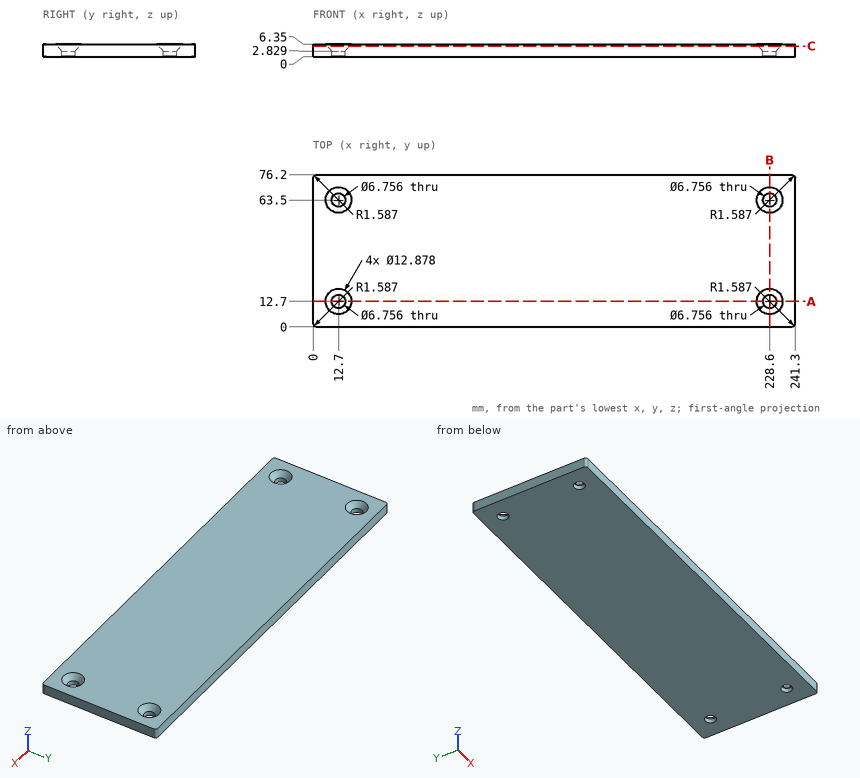
The drawing under review shows one solid part. Ordinate dimensions are in mm from its lowest x, y, z. Coordinates: 2 decimals unless noted, no trailing zeros. Write each loop counter-clockwise with the first axis right and the second up, starting at its lowest first coordinate (ties: lowest second). Pieces come first, ordered by that corner, then holes. Notation, with made-up numbers: (35.5, 37) -> (85.5, 37) arc R21 ccw to (85.5, 59) -> close; hole circle Ø3 at (-37, -26). An arc over 180 degrees is marked (long way). Write each question's results on one line, items separated by ' | '. Start each with the question number.
1) Wall thickness on L1, parallel to X at y = 63.5, z = 1.8; L2, parallel to X at y = 10.5, z = 1.25 (1 decimal); L3, parallel to Z at x = 225, y = 65: over which ranges is each line inside the solid? List them lowest first. Write a range as [from, to].
2) Consider section B-B (x = 228.6). Write out the cut boundary in (y, z).
3) Consider section C-C (z = 5.25). Write out the cut boundary in (x, y) (1 decimal).
4) Consider section A-A (y = 12.7). Write out the cut boundary in (x, z).
5) Insertion check: pin 1 (5.5 mm diameter, centred on x = 228.6, y = 12.7, fed in from -Z); pin 2 (9 mm diameter, centred on x = 12.7, y = 12.7, fed in from +Z). Each pin has a flat end and moves straight along its axis. Give the tip position at first contact, or say it passes through.
Geometry says:
1) L1: [0, 9.32], [16.08, 225.22], [231.98, 241.3] | L2: [0, 10.1], [15.3, 226], [231.2, 241.3] | L3: [0, 3.43]
2) outline: (0, 0) -> (9.32, 0) -> (9.32, 2.83) -> (6.26, 6.35) -> (0, 6.35) -> close; (16.08, 0) -> (60.12, 0) -> (60.12, 2.83) -> (57.06, 6.35) -> (19.14, 6.35) -> (16.08, 2.83) -> close; (66.88, 0) -> (76.2, 0) -> (76.2, 6.35) -> (69.94, 6.35) -> (66.88, 2.83) -> close
3) outline: (0, 1.6) arc R1.6 ccw to (1.6, 0) -> (239.7, 0) arc R1.6 ccw to (241.3, 1.6) -> (241.3, 74.6) arc R1.6 ccw to (239.7, 76.2) -> (1.6, 76.2) arc R1.6 ccw to (0, 74.6) -> close; hole circle Ø11 at (12.7, 12.7); hole circle Ø11 at (12.7, 63.5); hole circle Ø11 at (228.6, 12.7); hole circle Ø11 at (228.6, 63.5)
4) outline: (0, 0) -> (9.32, 0) -> (9.32, 2.83) -> (6.26, 6.35) -> (0, 6.35) -> close; (16.08, 0) -> (225.22, 0) -> (225.22, 2.83) -> (222.16, 6.35) -> (19.14, 6.35) -> (16.08, 2.83) -> close; (231.98, 0) -> (241.3, 0) -> (241.3, 6.35) -> (235.04, 6.35) -> (231.98, 2.83) -> close
5) pin 1: through | pin 2: z = 4.12
